from build123d import *

# Parameters (mm, degrees)
F1_DEPTH = 0.8
F2_R     = 0.4
F3_R     = 0.39999
F4_W     = 4.168279469
F4_H     = 8
F5_DEPTH = 0.4
F6_DEPTH = 0.4


# Not quite as in the source:
# - a fillet or chamfer is up to 0.001 mm smaller than in the source, because OpenCascade refuses the exact size


with BuildPart() as f1:
    # F0 (on Top) → F1 (new body)
    with BuildSketch(Plane.XY):
        with BuildLine():
            ThreePointArc((0, 38.1792416396), (-9.2970452561, 28.8821963835), (-12.7, 16.1821963835))
            ThreePointArc((-12.7, 16.1821963835), (-7.7676026835, 9.8183978835), (0, 7.6992416396))
            ThreePointArc((0, 7.6992416396), (7.7676026835, 9.8183978835), (12.7, 16.1821963835))
            ThreePointArc((12.7, 16.1821963835), (9.3014350381, 28.8847308253), (0, 38.1792416396))
        make_face()
    extrude(amount=F1_DEPTH)

    # F2
    f2_edges = [f1.edges().sort_by_distance(p)[0] for p in [
        (-9.297045, 28.882196, 0.8),
        (-7.767603, 9.818398, 0.8),
        (7.767603, 9.818398, 0.8),
        (9.301435, 28.884731, 0.8),
    ]]
    fillet(f2_edges, radius=F2_R)

    # F3 (radius 0.4 in the source; OpenCascade refuses exactly that, so slightly less here)
    f3_edges = [f1.edges().sort_by_distance(p)[0] for p in [
        (7.767603, 9.818398, 0),
        (9.301435, 28.884731, 0),
        (-7.767603, 9.818398, 0),
        (-9.297045, 28.882196, 0),
    ]]
    fillet(f3_edges, radius=F3_R)

    # F4 (on Top) + F1_face (on face) + F1_face1 (on face) → F5 (cut)
    with BuildSketch(Plane.XY):
        Polygon((1.9827442754, 19.357689971), (-4.0172557246, 19.357689971), (-1.0172557246, 14.1615375483), align=None)
        with BuildLine():
            Line((-9.0172557246, 19.357689971), (-9.0172557246, 15.857689971))
            ThreePointArc((-9.0172557246, 15.857689971), (-6.5423819904, 16.8828162368), (-5.5172557246, 19.357689971))
            Line((-5.5172557246, 19.357689971), (-9.0172557246, 19.357689971))
        make_face()
        Polygon((-1.0172557246, 25.5538423937), (-4.0172557246, 20.357689971), (1.9827442754, 20.357689971), align=None)
        with Locations((5.56688401, 15.357689971)):
            Rectangle(F4_W, F4_H)
        with BuildLine():
            Line((-9.0172557246, 20.357689971), (-5.5172557246, 20.357689971))
            ThreePointArc((-5.5172557246, 20.357689971), (-6.5423819904, 22.8325637051), (-9.0172557246, 23.857689971))
            Line((-9.0172557246, 23.857689971), (-9.0172557246, 20.357689971))
        make_face()
        with Locations((5.56688401, 24.357689971)):
            Rectangle(F4_W, F4_H)
    with BuildSketch(Plane(origin=(0.0014081173, 21.2624606857, 0.8), x_dir=(1, 0, 0), z_dir=(0, 0, 1))):
        with BuildLine():
            ThreePointArc((-0.0012370935, 16.4537632815), (-8.9926932828, 7.3490618207), (-12.3013148115, -5.0119614651))
            ThreePointArc((-12.3013148115, -5.0119614651), (-7.5186387645, -11.1302175722), (-0.0238816927, -13.1638508721))
            add(Edge.make_bspline(
                [(-0.0238816927, -13.1638508721), (-0.0125655835, -13.1632140826), (-0.0014081173, -13.1622533084), (0.009749349, -13.1632140826), (0.0210654582, -13.1638508721)],
                knots=[0, 0, 0, 0, 0, 1, 1, 1, 1, 1], degree=4))
            ThreePointArc((0.0210654582, -13.1638508721), (7.5158860187, -11.1301754171), (12.2985497378, -5.0118178891))
            ThreePointArc((12.2985497378, -5.0118178891), (8.9943044567, 7.3515302466), (-0.0012370935, 16.4537632815))
        make_face()
    with BuildSketch(Plane(origin=(0.001408117, 21.262461098, 0), x_dir=(1, 0, 0), z_dir=(0, 0, -1))):
        with BuildLine():
            ThreePointArc((12.2985597415, 5.0118200202), (7.5158922747, 11.1301836793), (0.0210648966, 13.1638612686))
            add(Edge.make_bspline(
                [(0.0210648966, 13.1638612686), (0.0097490703, 13.1632244951), (-0.001408117, 13.1622637449), (-0.0125653043, 13.1632244951), (-0.0238811306, 13.1638612686)],
                knots=[0, 0, 0, 0, 0, 1, 1, 1, 1, 1], degree=4))
            ThreePointArc((-0.0238811306, 13.1638612686), (-7.5186450215, 11.1302258334), (-12.301324816, 5.0119635927))
            ThreePointArc((-12.301324816, 5.0119635927), (-8.9927009274, -7.3490681805), (-0.0012370975, -16.4537744762))
            ThreePointArc((-0.0012370975, -16.4537744762), (8.9943121009, -7.3515366081), (12.2985597415, 5.0118200202))
        make_face()
    extrude(amount=-F5_DEPTH, dir=(0, 0, 1), mode=Mode.SUBTRACT)

    # F4 (on Top) → F6 (join)
    with BuildSketch(Plane.XY):
        with BuildLine():
            Line((-9.0172557246, 19.357689971), (-9.0172557246, 15.857689971))
            ThreePointArc((-9.0172557246, 15.857689971), (-6.5423819904, 16.8828162368), (-5.5172557246, 19.357689971))
            Line((-5.5172557246, 19.357689971), (-9.0172557246, 19.357689971))
        make_face()
        with BuildLine():
            Line((-9.0172557246, 20.357689971), (-5.5172557246, 20.357689971))
            ThreePointArc((-5.5172557246, 20.357689971), (-6.5423819904, 22.8325637051), (-9.0172557246, 23.857689971))
            Line((-9.0172557246, 23.857689971), (-9.0172557246, 20.357689971))
        make_face()
        Polygon((-1.0172557246, 25.5538423937), (-4.0172557246, 20.357689971), (1.9827442754, 20.357689971), align=None)
        Polygon((1.9827442754, 19.357689971), (-4.0172557246, 19.357689971), (-1.0172557246, 14.1615375483), align=None)
        with Locations((5.56688401, 24.357689971)):
            Rectangle(F4_W, F4_H)
        with Locations((5.56688401, 15.357689971)):
            Rectangle(F4_W, F4_H)
    extrude(amount=-F6_DEPTH)


solid = f1.part
CAD build for the part. Positions are in the model's coordinates, mm. A direction names the side the tool comes from. Round coordinates to 2 decimals unless told otherwise and drop trailing zeros. Write each loop counter-clockwise with the first axis right and the second up, starting at its lowest first coordinate (ties: lowest second). Pieces come first, ordered by that corner, then holes. Notation, with made-up numbers: M 60,-2.75 L 109,-2.75 A10 cw 109,9.25 Z; hole C 65,-35.5 d10. An arc over 180 degrees is marked long. Use a Markdown table: item, result. Add a question column.
1. 3-axis set-ups, long thin cutter, end or side, ignore diameter. For faces 3 (the face through (0, 20, 0.4)), 4 (the face through (-6.52, 22.81, -0.2)), 5 (the face through (-6.57, 16.856, -0.197)): which of +Z, -Z, +X, -X, +Y, -Y reach the whole face in a straight line?
2. Pull direction X, two halves, no side cores. Call faces 1 (the face through (-8, 18, -0.4)), 2 (the face through (0.46, 16.72, -0.2)): released by +X, released by -X, zero draft, split by the parting line, or undercut.
3. Drill centre lines: probe 1 along Z at (x, y) = (10.5, 24.5); probe 2 along X at (y, z) = (28, -0.1); probe 3 along Y at (x, z) = (5, 0.7). Where is each one in solid material? Low to high.
4. Flat gauge pins, fed straight in: P1, Ø3, axis at x = 0.5, y = 32.5, coming from the -Z side; P2, Ø4, axis at x = 0.5, y = 32.5, coming from the +Z side. Where does each tip first touch, or does it go through?
5. Slice it at A-A on z = -0.2. Give the cut face in (x, y), then the cut area to 3 significant figures.
Reply:
| question | item | result |
|---|---|---|
| 1 | face 3 | +Z |
| 1 | face 4 | -Z, +Y |
| 1 | face 5 | -Z, -Y |
| 2 | face 1 | zero draft |
| 2 | face 2 | undercut |
| 3 | probe 1 | z = 0 to 0.4 |
| 3 | probe 2 | x = 3.48 to 7.65 |
| 3 | probe 3 | y = 8.57 to 8.85, 33.84 to 34.22 |
| 4 | P1 | stops at z = 0 |
| 4 | P2 | stops at z = 0.4 |
| 5 | outline | M -9.02,15.86 A3.5 ccw -5.52,19.36 L -9.02,19.36 Z; M -9.02,20.36 L -5.52,20.36 A3.5 ccw -9.02,23.86 Z; M -4.02,19.36 L -1.02,14.16 L 1.98,19.36 Z; M -4.02,20.36 L 1.98,20.36 L -1.02,25.55 Z; M 3.48,11.36 L 7.65,11.36 L 7.65,19.36 L 3.48,19.36 Z; M 3.48,20.36 L 7.65,20.36 L 7.65,28.36 L 3.48,28.36 Z |
| 5 | area | 117 mm^2 |
